Answer from the drawing. Dimensions are ordinates in mm from the lowest x, y and z of the part. Give positions to 0.01 mm unless a question says otherwise; leave off trailing zeros. Loops run counter-clockwise (first coordinate to the right, second up) from the corner with the lowest first, then second, coordinate; pieces in that order, holes last. Notation, with made-up numbers: (51, 61.25) - (88, 61.25) arc R6 ccw to (88, 72.25) - close; hole circle Ø9 at (-25.75, 56). An arc over 180 degrees is marked (long way). One line per question, with ' | ' between items. Start each with the question number.
1. Section A-A (x = 52) is taken. Determine the outline of the cut face in (y, z), plus the area to 3 significant figures.
2. Section D-D (x = 97.5) is taken. Determine the outline of the cut face in (y, z).
3. Section B-B (z = 2.5) is taken. Determine the outline of the cut face in (x, y) (3 decimals).
4. Section C-C (y = 13) is taken. Determine the outline of the cut face in (x, z).
5. Each of these flat-tipped pins is pushed along its axis until it touches: pin 1 (1 mm diameter, centred on x = 86, z = 3, fed in from +Y); pin 2 (2.5 mm diameter, centred on y = 42, z = 3.5, fed in from +X); pin 3 (2 mm diameter, centred on y = 15.5, z = 0.5, fed in from +X). Where does it stop, or does it pass through?
6. Find the intervals of material crossed by line 1 (Y direction, x = 52, z = 3.9); line 2 (X direction, y = 43, z = 0.45); line 3 (X direction, y = 47, z = 2.1), in increasing order.
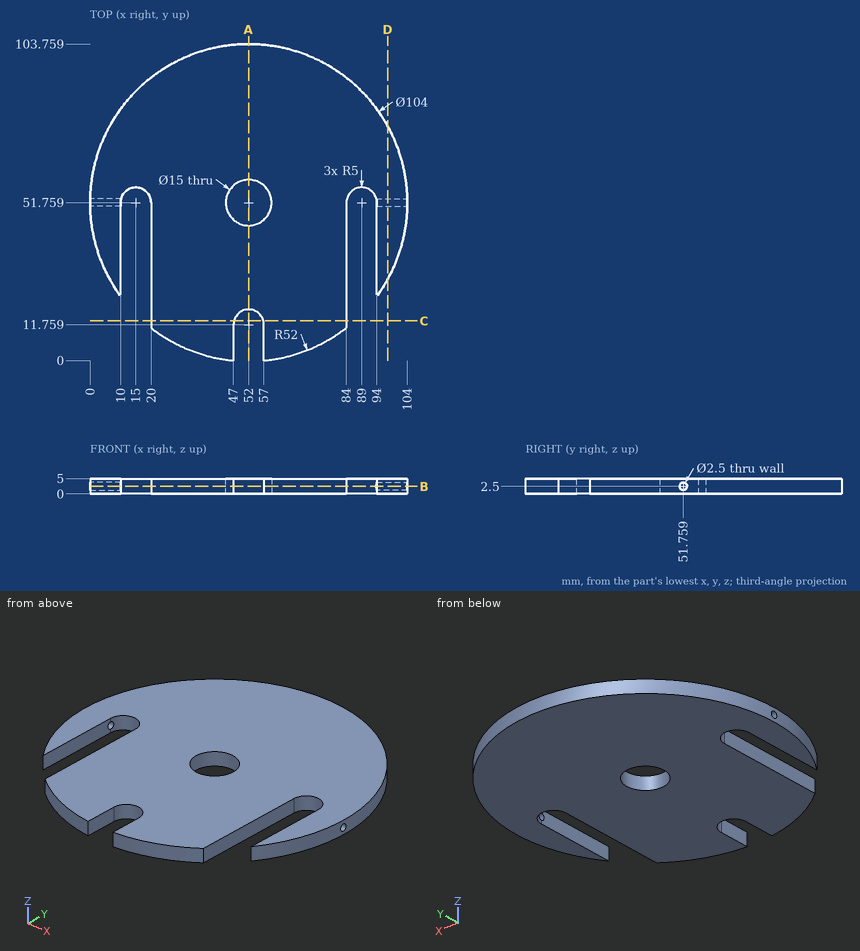
Conclusion:
1) outline: (16.76, 0) - (44.26, 0) - (44.26, 5) - (16.76, 5) - close; (59.26, 0) - (103.76, 0) - (103.76, 5) - (59.26, 5) - close | area: 360 mm²
2) outline: (26.58, 0) - (76.93, 0) - (76.93, 5) - (26.58, 5) - close; hole circle Ø2.5 at (51.76, 2.5)
3) outline: (0.015, 50.509) arc R52 ccw to (10, 21.1) - (10, 50.509) - close; (0.015, 53.009) - (10.159, 53.009) arc R5 cw to (20, 51.759) - (20, 10.771) arc R52 ccw to (47, 0) - (47, 11.759) arc R5 cw to (57, 11.759) - (57, 0) arc R52 ccw to (84, 10.771) - (84, 51.759) arc R5 cw to (93.841, 53.009) - (103.985, 53.009) arc R52 ccw to start; (94, 21.1) arc R52 ccw to (103.985, 50.509) - (94, 50.509) - close; hole circle Ø15 at (52, 51.759)
4) outline: (20, 0) - (47.16, 0) - (47.16, 5) - (20, 5) - close; (56.84, 0) - (84, 0) - (84, 5) - (56.84, 5) - close
5) pin 1: y = 91.53 | pin 2: x = 103.3 | pin 3: x = 84
6) line 1: 16.76 to 44.26, 59.26 to 103.76 | line 2: 0.74 to 10, 20 to 84, 94 to 103.26 | line 3: 0.22 to 10, 20 to 46.2, 57.8 to 84, 94 to 103.78
